Autodesk Inventor part; units mm, degrees
ref_plane "YZ Plane" through (0, 0, 0) normal (1, 0, 0) x (0, 1, 0)
ref_plane "XZ Plane" through (0, 0, 0) normal (0, 1, 0) x (-1, 0, 0)
ref_plane "XY Plane" through (0, 0, 0) normal (0, 0, 1) x (1, 0, 0)
sketch "Sketch1" plane through (0, 0, 0) normal (0, 1, 0) x (-1, 0, 0)
  line L0 (0, 0) -> (10.2, 0)
  line L1 (10.2, 0) -> (10.2, -25.4)
  line L2 (10.2, -25.4) -> (0, -25.4)
  line L3 (0, -25.4) -> (0, 0)
  dimension "d0" = 10.2
  dimension "d1" = 25.4
extrude "Extrusion1" add sketch "Sketch1" along normal blind 1
sketch "Sketch2" plane through (0, 0, 0) normal (0, -1, 0) x (1, 0, 0)
  line L0 (-10.2, -25.4) -> (-10.2, 0)
  line L1 (-10.2, 0) -> (-5.1, 0)
  line L2 (-10.2, 0) -> (0, 0)
  line L3 (-5.1, 0) -> (-5.1, -25.4)
  line L4 (0, -25.4) -> (-10.2, -25.4)
  line L5 (-5.1, -22.7265) -> (-1.29, -22.7265)
  line L6 (-1.29, -22.7265) -> (-1.29, 0)
  line L7 (-1.29, 0) -> (-1.29, -2.54)
  circle A0 centre (-1.29, -2.54) radius 0.5
  line L8 (-1.29, -2.54) -> (-1.29, -5.08)
  line L9 (-1.29, -5.08) -> (-1.29, -7.62)
  line L10 (-1.29, -7.62) -> (-1.29, -10.16)
  line L11 (-1.29, -10.16) -> (-1.29, -12.7)
  line L12 (-1.29, -12.7) -> (-1.29, -15.24)
  line L13 (-1.29, -15.24) -> (-1.29, -17.78)
  line L14 (-1.29, -17.78) -> (-1.29, -20.32)
  line L15 (-1.29, -20.32) -> (-1.29, -22.86)
  circle A1 centre (-1.29, -5.08) radius 0.5
  circle A2 centre (-1.29, -7.62) radius 0.5
  circle A3 centre (-1.29, -10.16) radius 0.5
  circle A4 centre (-1.29, -12.7) radius 0.5
  circle A5 centre (-1.29, -15.24) radius 0.5
  circle A6 centre (-1.29, -17.78) radius 0.5
  circle A7 centre (-1.29, -20.32) radius 0.5
  circle A8 centre (-1.29, -22.86) radius 0.5
  circle A9 centre (-8.91, -2.54) radius 0.5
  circle A10 centre (-8.91, -5.08) radius 0.5
  circle A11 centre (-8.91, -7.62) radius 0.5
  circle A12 centre (-8.91, -10.16) radius 0.5
  circle A13 centre (-8.91, -12.7) radius 0.5
  circle A14 centre (-8.91, -15.24) radius 0.5
  circle A15 centre (-8.91, -17.78) radius 0.5
  circle A16 centre (-8.91, -20.32) radius 0.5
  circle A17 centre (-8.91, -22.86) radius 0.5
  circle A18 centre (-1.29, -22.86) radius 0.225
  circle A19 centre (-1.29, -20.32) radius 0.225
  circle A20 centre (-1.29, -17.78) radius 0.225
  circle A21 centre (-1.29, -15.24) radius 0.225
  circle A22 centre (-1.29, -12.7) radius 0.225
  circle A23 centre (-1.29, -10.16) radius 0.225
  circle A24 centre (-1.29, -7.62) radius 0.225
  circle A25 centre (-1.29, -5.08) radius 0.225
  circle A26 centre (-1.29, -2.54) radius 0.225
  circle A27 centre (-8.91, -22.86) radius 0.225
  circle A28 centre (-8.91, -20.32) radius 0.225
  circle A29 centre (-8.91, -17.78) radius 0.225
  circle A30 centre (-8.91, -15.24) radius 0.225
  circle A31 centre (-8.91, -12.7) radius 0.225
  circle A32 centre (-8.91, -10.16) radius 0.225
  circle A33 centre (-8.91, -7.62) radius 0.225
  circle A34 centre (-8.91, -5.08) radius 0.225
  circle A35 centre (-8.91, -2.54) radius 0.225
  dimension "d4" = 5.1
  dimension "d5" = 90
  dimension "d6" = 3.81
  dimension "d7" = 2.54
  dimension "d8" = 1
  dimension "d9" = 2.54
  dimension "d10" = 2.54
  dimension "d11" = 2.54
  dimension "d12" = 2.54
  dimension "d13" = 2.54
  dimension "d14" = 2.54
  dimension "d15" = 2.54
  dimension "d16" = 2.54
  dimension "d17" = 1
  dimension "d18" = 1
  dimension "d19" = 1
  dimension "d20" = 1
  dimension "d21" = 1
  dimension "d22" = 1
  dimension "d23" = 1
  dimension "d24" = 1
  dimension "d27" = 0.45
  dimension "d28" = 0.45
  dimension "d29" = 0.45
  dimension "d30" = 0.45
  dimension "d31" = 0.45
  dimension "d32" = 0.45
  dimension "d33" = 0.45
  dimension "d34" = 0.45
  dimension "d35" = 0.45
extrude "Extrusion3" add sketch "Sketch2" along normal blind 3.5 contours A18 L6 L5 | L5 L6 A18 | A26 L6 | L6 A26 | A19 L6 | L6 A19 | A25 L6 | L6 A25 | A20 L6 | L6 A20 | A24 L6 | L6 A24 | A21 L6 | L6 A21 | A23 L6 | L6 A23 | A22 L6 | L6 A22 | A27 | A28 | A29 | A30 | A31 | A32 | A33 | A34 | A35
sketch "Sketch3" plane through (0, 0, 0) normal (0, -1, 0) x (1, 0, 0)
  circle A0 centre (-8.91, -22.86) radius 0.225
  circle A1 centre (-8.91, -22.86) radius 0.5
  circle A2 centre (-8.91, -20.32) radius 0.225
  circle A3 centre (-8.91, -20.32) radius 0.5
  circle A4 centre (-8.91, -17.78) radius 0.225
  circle A5 centre (-8.91, -17.78) radius 0.5
  circle A6 centre (-8.91, -15.24) radius 0.225
  circle A7 centre (-8.91, -15.24) radius 0.5
  circle A8 centre (-8.91, -12.7) radius 0.225
  circle A9 centre (-8.91, -12.7) radius 0.5
  circle A10 centre (-8.91, -10.16) radius 0.225
  circle A11 centre (-8.91, -10.16) radius 0.5
  circle A12 centre (-8.91, -7.62) radius 0.225
  circle A13 centre (-8.91, -7.62) radius 0.5
  circle A14 centre (-8.91, -5.08) radius 0.225
  circle A15 centre (-8.91, -5.08) radius 0.5
  circle A16 centre (-8.91, -2.54) radius 0.225
  circle A17 centre (-8.91, -2.54) radius 0.5
  circle A18 centre (-1.29, -22.86) radius 0.225
  circle A19 centre (-1.29, -22.86) radius 0.5
  circle A20 centre (-1.29, -20.32) radius 0.225
  circle A21 centre (-1.29, -20.32) radius 0.5
  circle A22 centre (-1.29, -17.78) radius 0.225
  circle A23 centre (-1.29, -17.78) radius 0.5
  circle A24 centre (-1.29, -15.24) radius 0.225
  circle A25 centre (-1.29, -15.24) radius 0.5
  circle A26 centre (-1.29, -12.7) radius 0.225
  circle A27 centre (-1.29, -12.7) radius 0.5
  circle A28 centre (-1.29, -10.16) radius 0.225
  circle A29 centre (-1.29, -10.16) radius 0.5
  circle A30 centre (-1.29, -7.62) radius 0.225
  circle A31 centre (-1.29, -7.62) radius 0.5
  circle A32 centre (-1.29, -5.08) radius 0.225
  circle A33 centre (-1.29, -5.08) radius 0.5
  circle A34 centre (-1.29, -2.54) radius 0.225
  circle A35 centre (-1.29, -2.54) radius 0.5
  point P0 (0, 0)
  dimension "d38" = 1
  dimension "d39" = 1
  dimension "d40" = 1
  dimension "d41" = 1
  dimension "d42" = 1
  dimension "d43" = 1
  dimension "d44" = 1
  dimension "d45" = 1
  dimension "d46" = 1
  dimension "d47" = 1
  dimension "d48" = 1
  dimension "d49" = 1
  dimension "d50" = 1
  dimension "d51" = 1
  dimension "d52" = 1
  dimension "d53" = 1
  dimension "d54" = 1
  dimension "d55" = 1
extrude "Extrusion4" add sketch "Sketch3" along normal blind 0.1 contours A0 | A1 | A2 | A3 | A4 | A5 | A6 | A7 | A8 | A9 | A10 | A11 | A12 | A13 | A14 | A15 | A16 | A17 | A18 | A19 | A20 | A21 | A22 | A23 | A24 | A25 | A26 | A27 | A28 | A29 | A30 | A31 | A32 | A33 | A34 | A35
sketch "Sketch5" plane through (0, 1, 0) normal (0, 1, 0) x (1, 0, 0)
  line L0 (0, 0) -> (0, 25.4)
  line L1 (0, 0) -> (0, 12.7)
  line L2 (0, 12.7) -> (-5.1, 12.7)
  line L3 (-6.69, 0) -> (-6.69, 25.4)
  line L4 (-6.69, 25.4) -> (-3.51, 25.4)
  line L5 (-3.51, 25.4) -> (-3.51, 0)
  line L6 (-3.51, 0) -> (-6.69, 0)
  line L7 (-6.69, 0) -> (-3.51, 25.4) construction
  line L8 (-6.69, 25.4) -> (-3.51, 0) construction
  dimension "d61" = 12.7
  dimension "d62" = 5.1
  dimension "d63" = 3.18
extrude "Extrusion5" add sketch "Sketch5" along normal blind 0.2
sketch "Sketch6" plane through (0, 1.2, 0) normal (0, 1, 0) x (1, 0, 0)
  line L0 (0, 0) -> (0, 12.7)
  line L1 (0, 0) -> (0, 25.4)
  line L2 (0, 12.7) -> (-5.1, 12.7)
  line L3 (-6.1, 0) -> (-6.1, 25.4)
  line L4 (-6.1, 25.4) -> (-4.1, 25.4)
  line L5 (-4.1, 25.4) -> (-4.1, 0)
  line L6 (-4.1, 0) -> (-6.1, 0)
  line L7 (-6.1, 0) -> (-4.1, 25.4) construction
  line L8 (-6.1, 25.4) -> (-4.1, 0) construction
  dimension "d66" = 12.7
  dimension "d67" = 5.1
  dimension "d68" = 2
extrude "Extrusion6" add sketch "Sketch6" along normal blind 1.4
properties part number "Detector"
Verification items for the finished model (mm, model axes). A direction names the side the tool comes from. Give positions to 0.01 mm unless a question says otherwise; leave off trailing zeros. Order: outer loops, then holes, each group sorted by start corner. A loop starts at its lowest first (then second) coordinate and runs counter-clockwise, first axis right, second up. Notation, with made-up numbers: (49.25, 81) - (89.25, 81) arc R18 cw to (89.25, 94) - close; hole circle Ø7 at (26, 24.5). An arc over 180 degrees is marked (long way). Answer as CSV lines item,"result". Start each with the question number.
Item 1: Access from +Z, -Z, +X, -X, +Y, -Y to the whole of each face (thin tool, end or side, straight path). Record for faces 1 (the face through (-2, 1, -13)), 2 (the face through (-8, 1, -13)), 3 (the face through (-5, 2.6, -13)).
Item 2: Gauge pin test, flat ends, axial feed: pin 1 (3 mm diameter, centred on y = -2, z = -3.5, fed in from +X) (3 decimals); pin 2 (0.5 mm diameter, centred on x = -6.5, z = -13.5, fed in from +Y); pin 3 (1.8 mm diameter, centred on x = -2.5, z = -12, fed in from +Y). Record the tip position at first contact, or that the pin passes through.
Item 3: Section check A-A, the plane y = -2.25. State how many separate pieces and enclosed holes the cut face has, plus the area to 3 significant figures.
Item 4: Section check B-B, the plane z = -19. Record the boundary of the cut face in (x, y).
Item 5: Section check D-D, the plane y = 2.25. Record the boundary of the cut face in (x, z).
Item 6: Material ranges on L1, parallel to Y at x = -1.5, z = -13.5; L2, parallel to X at y = 2.5, z = -23; L3, parallel to Y at x = -4, z = -17.5, recorded low to high.
Item 7: Section check C-C, the plane x = -2.75. Record the boundary of the cut face in (y, z), plus the area to 3 significant figures.
Filled in:
1,face 1,"+Z, -Z, +X, +Y"
1,face 2,"+Z, -Z, -X, +Y"
1,face 3,"+Z, -Z, +X, -X, +Y"
2,pin 1,"x = -1.065"
2,pin 2,"y = 1.2"
2,pin 3,"y = 1"
3,separate pieces,"18"
3,enclosed holes,"0"
3,area,"2.86 mm^2"
4,outline,"(-10.2, 0) - (0, 0) - (0, 1) - (-3.51, 1) - (-3.51, 1.2) - (-4.1, 1.2) - (-4.1, 2.6) - (-6.1, 2.6) - (-6.1, 1.2) - (-6.69, 1.2) - (-6.69, 1) - (-10.2, 1) - close"
5,outline,"(-6.1, -25.4) - (-4.1, -25.4) - (-4.1, 0) - (-6.1, 0) - close"
6,L1,"0 to 1"
6,L2,"-6.1 to -4.1"
6,L3,"0 to 1.2"
7,outline,"(0, -25.4) - (1, -25.4) - (1, 0) - (0, 0) - close"
7,area,"25.4 mm^2"
